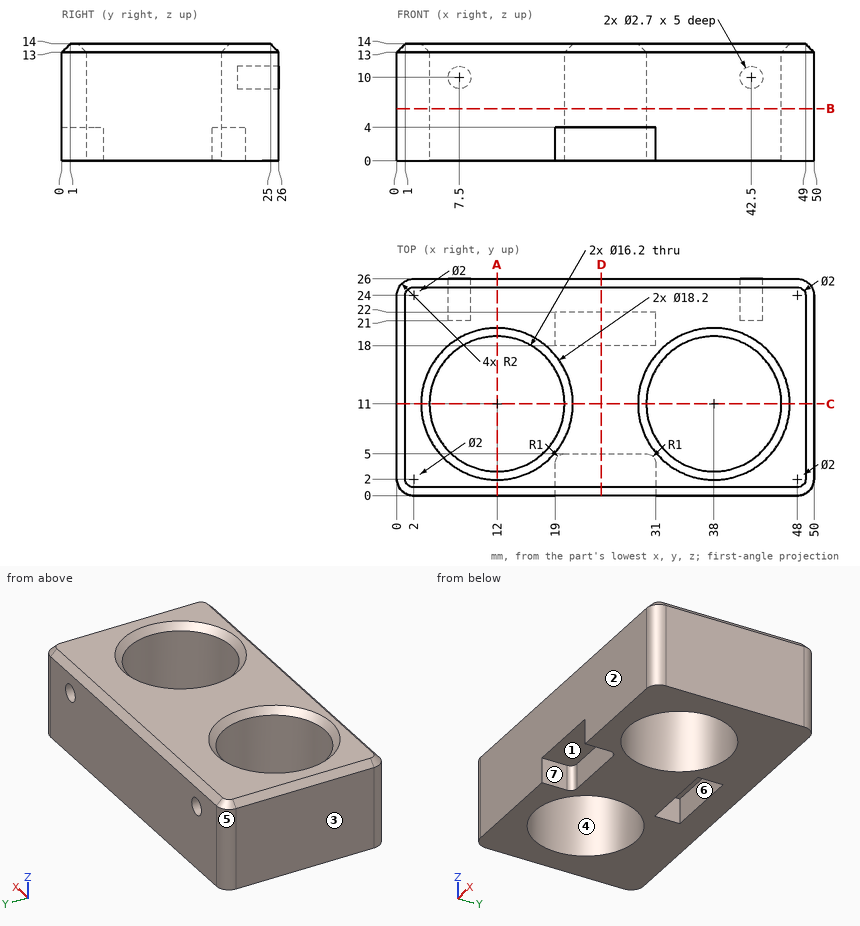
Part print with two shaded views. Sizes in mm from the minimum x, y, z corner. A direction names the side the tool comes from. Round coordinates to 2 decimals unless told otherwise and drop trailing zeros. Order: outer loops, then holes, each group sorted by start corner. A loop starts at its lowest first (then second) coordinate and runs counter-clockwise, first axis right, second up. Notation, with made-up numbers: M 14,-18 L 42,-18 A16 cw 42,9 Z; hole C 74,19 d10. An arc over 180 degrees is marked long. Answer in a Markdown table with one row per item. Add a question column.
Q1. Cut at D-D on x = 24.5. Give the cut face in (y, z), and give its area (3 significant figures).
Q2. Cut at A-A on x = 12. Give the cut face in (y, z).
Q3. 3-axis set-ups, long thin cutter, end or side, ignore diameter. For the marked faces 5, 6 and 7: which of +Z, -Z, +X, -X, +Y, -Y reach the whole face in a straight line?
Q4. Pin check, flat tips, straight feed: pin 1 (1.2 mm diameter, centred on x = 27, z = 1.5, fed in from -Y); pin 2 (1.2 mm diameter, centred on y = 1.5, z = 1.5, fed in from +X); pin 3 (2.5 mm diameter, centred on x = 42.5, z = 10, fed in from +Y). Stop position of each tip, or through.
Q5. Wall check: L1, parallel to Z at x = 42.5, y = 24.25; L2, parallel to Y at x = 12, z = 3; L3, parallel to X at y = 18.5, z = 7.5. Give the ranges that are in metal, low to high. Write a range as from..to.
Q6. Cut at C-C on y = 11. Give the cut face in (x, z).
Q7. Cut at B-B on z = 6.25. Give the cut face in (x, y).
Q8. Mould opens along X. For the marked faces 1, 2, 3 and 4 say: +X half, -X half, draft (parallel to the pull), parting line (faces both ways), or undercut.
Established:
| question | item | result |
|---|---|---|
| 1 | outline | M 0,4 L 5,4 L 5,0 L 18,0 L 18,4 L 22,4 L 22,0 L 26,0 L 26,13 L 25,14 L 1,14 L 0,13 Z |
| 1 | area | 327 mm2 |
| 2 | outline | M 0,0 L 2.9,0 L 2.9,13 L 1.9,14 L 1,14 L 0,13 Z; M 19.1,0 L 26,0 L 26,13 L 25,14 L 20.1,14 L 19.1,13 Z |
| 3 | face 5 | +Z, -Z, -X, +Y |
| 3 | face 6 | -Z |
| 3 | face 7 | -Z, -Y |
| 4 | pin 1 | stops at y = 5 |
| 4 | pin 2 | stops at x = 50 |
| 4 | pin 3 | stops at y = 21 |
| 5 | L1 | z = 0..8.65, 11.35..14 |
| 5 | L2 | y = 0..2.9, 19.1..26 |
| 5 | L3 | x = 0..8.94, 15.06..34.94, 41.06..50 |
| 6 | outline | M 0,0 L 3.9,0 L 3.9,13 L 2.9,14 L 1,14 L 0,13 Z; M 20.1,0 L 29.9,0 L 29.9,13 L 28.9,14 L 21.1,14 L 20.1,13 Z; M 46.1,0 L 50,0 L 50,13 L 49,14 L 47.1,14 L 46.1,13 Z |
| 7 | outline | M 0,2 A2 ccw 2,0 L 48,0 A2 ccw 50,2 L 50,24 A2 ccw 48,26 L 2,26 A2 ccw 0,24 Z; hole C 12,11 d16.2; hole C 38,11 d16.2 |
| 8 | face 1 | undercut |
| 8 | face 2 | draft |
| 8 | face 3 | -X half |
| 8 | face 4 | undercut |
